Geometry: final body of the model. Coordinates: model frame, mm. Face numbers are marked on the shaded views. A direction names the side the tool comes from. Round coordinates to 2 decimals unless told otherwise and drop trailing zeros. Loops run counter-clockwise (first coordinate to the right, second up) from the corner with the lowest first, then second, coordinate; pieces in that order, holes last. Notation, with made-up numbers: M 57.25,53.25 L 111.25,53.25 A4 ccw 111.25,58.25 Z; hole C -12,14 d8. An arc over 180 degrees is marked long. Write each question's results on one line, items separated by ' | '.
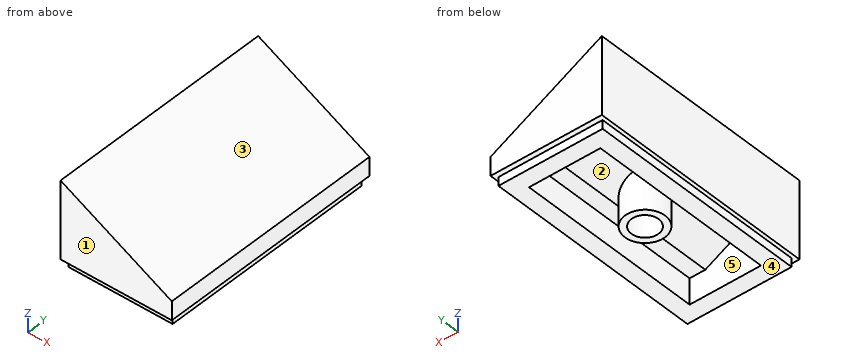
Solid Edge part; units mm, degrees
sketch "Sketch1" plane through (0, 0, 0) normal (0, 0, 1) x (1, 0, 0)
  line L0 (3.9, 7.9) -> (-3.9, 7.9)
  line L1 (-3.9, 7.9) -> (-3.9, -7.9)
  line L2 (-3.9, -7.9) -> (3.9, -7.9)
  line L3 (3.9, -7.9) -> (3.9, 7.9)
extrude "Protrusion1" add sketch "Sketch1" along normal blind 6
sketch "Sketch2" plane through (0, -7.9, 3) normal (0, -1, 0) x (1, 0, 0)
  line L0 (3.9, -3) -> (3.9, -1.1)
  line L1 (3.9, -1.1) -> (-3.9, 3)
  line L2 (-3.9, 3) -> (-3.9, 3.5621)
  line L3 (-3.9, 3.5621) -> (6.8698, 3.4105)
  line L4 (6.8698, 3.4105) -> (3.9, -3)
extrude "ExtrudedCutout_1" cut sketch "Sketch2" against normal blind 28.4067
sketch "Sketch3" plane through (0, 0, 0) normal (0, 0, -1) x (1, 0, 0)
  line L0 (3.65, 7.65) -> (-3.65, 7.65)
  line L1 (-3.65, 7.65) -> (-3.65, -7.65)
  line L2 (-3.65, -7.65) -> (3.65, -7.65)
  line L3 (3.65, -7.65) -> (3.65, 7.65)
  line L4 (-4.59, -8.7889) -> (5.3032, -8.7889)
  line L5 (5.3032, -8.7889) -> (5.3032, 8.7889)
  line L6 (5.3032, 8.7889) -> (-4.59, 8.7889)
  line L7 (-4.59, 8.7889) -> (-4.59, -8.7889)
extrude "ExtrudedCutout_2" cut sketch "Sketch3" against normal blind 0.6
sketch "Sketch4" plane through (0, 0, 0) normal (0, 0, -1) x (1, 0, 0)
  line L0 (-2.5, -6.5) -> (2.5, -6.5)
  line L1 (2.5, -6.5) -> (2.5, 6.5)
  line L2 (2.5, 6.5) -> (-2.5, 6.5)
  line L3 (-2.5, 6.5) -> (-2.5, -6.5)
extrude "ExtrudedCutout_3" cut sketch "Sketch4" against normal blind 1.8
sketch "Sketch5" plane through (0, 6.5, 0.9) normal (0, -1, 0) x (1, 0, 0)
  line L0 (-2.5, 0.9) -> (-2.5, 2.95)
  line L1 (1.4, 0.9) -> (-2.5, 2.95)
  line L2 (-2.5, 0.9) -> (1.4, 0.9)
extrude "Cutout1" cut sketch "Sketch5" along normal up to vertex (13 mm away)
sketch "Sketch6" plane through (0, 0, 0) normal (0, 0, -1) x (1, 0, 0)
  circle A0 centre (0, 0) radius 1.4
  circle A1 centre (0, 0) radius 0.95
extrude "ExtrudedProtrusion_2" add sketch "Sketch6" against normal blind 6.3788
sketch "Sketch7" plane through (0, -7.9, 3.3) normal (0, -1, 0) x (1, 0, 0)
  line L0 (-3.9, 2.7) -> (3.9, -1.4)
  line L1 (3.9, -1.4) -> (3.4688, 3.9064)
  line L2 (3.4688, 3.9064) -> (-3.9, 2.7)
extrude "ExtrudedCutout_5" cut sketch "Sketch7" against normal blind 34.0923
sketch "Sketch8" plane through (0, -7.9, 3.3) normal (0, -1, 0) x (0, 0, 1)
  line L0 (-2.7, -3.9) -> (-2.7, 3.9)
  line L1 (-2.7, 3.9) -> (2.7, 3.9)
  line L2 (2.7, 3.9) -> (-1.4, -3.9)
  line L3 (-1.4, -3.9) -> (-2.7, -3.9)
extrude "ExtrudedProtrusion_3" add sketch "Sketch8" along normal blind 0.1
sketch "Sketch9" plane through (0, 7.9, 3.3) normal (0, 1, 0) x (0, 0, -1)
  line L0 (-2.7, 3.9) -> (2.7, 3.9)
  line L1 (2.7, 3.9) -> (2.7, -3.9)
  line L2 (2.7, -3.9) -> (1.4, -3.9)
  line L3 (1.4, -3.9) -> (-2.7, 3.9)
extrude "ExtrudedProtrusion_4" add sketch "Sketch9" along normal blind 0.1
1. Section A-A (y = -5.75). Output: boundary loops of the cut face in (x, z), then the cut area to 3 significant figures.
Answer key:
outline: M -3.9,0.6 L -3.65,0.6 L -3.65,0 L -2.5,0 L -2.5,3.85 L 1.4,1.8 L 2.5,1.8 L 2.5,0 L 3.65,0 L 3.65,0.6 L 3.9,0.6 L 3.9,1.9 L -3.9,6 Z | area: 17.5 mm²
2. Section D-D (x = -0.5). Output: boundary loops of the cut face in (y, z).
Answer key:
outline: M -8,0.6 L -7.65,0.6 L -7.65,0 L -6.5,0 L -6.5,2.8 L -1.31,2.8 L -1.31,0 L -0.81,0 L -0.81,2.8 L 0.81,2.8 L 0.81,0 L 1.31,0 L 1.31,2.8 L 6.5,2.8 L 6.5,0 L 7.65,0 L 7.65,0.6 L 8,0.6 L 8,4.21 L -8,4.21 Z
3. Access query for the marked faces 4 and 5. Directions: +Z, -Z, +X, -X, +Y, -Y. A direction counts if a zero-diameter tool reaches every point of the face in a straight line with its end or side. Return the directions, or none.
Answer key:
face 4: -Z, +X, -X, +Y, -Y | face 5: -Z
4. Ray query, probe 1 along X at (y, z) = (0, 1.65); probe 2 along Y at (x, z) = (0, 1.5); probe 3 along Y at (x, z) = (-1.5, 1.4). Return the intervals inside material, ascending.
Answer key:
probe 1: x = -3.9 to -2.5, -1.4 to -0.95, 0.95 to 1.4, 2.5 to 3.9 | probe 2: y = -8 to -6.5, -1.4 to -0.95, 0.95 to 1.4, 6.5 to 8 | probe 3: y = -8 to -6.5, 6.5 to 8
5. Section C-C (z = 4.1). Output: boundary loops of the cut face in (x, y).
Answer key:
outline: M -3.9,-8 L -0.29,-8 L -0.29,8 L -3.9,8 Z
6. Section B-B (x = 0.75). Output: boundary loops of the cut face in (y, z).
Answer key:
outline: M -8,0.6 L -7.65,0.6 L -7.65,0 L -6.5,0 L -6.5,2.14 L -1.18,2.14 L -1.18,0 L -0.58,0 L -0.58,2.14 L 0.58,2.14 L 0.58,0 L 1.18,0 L 1.18,2.14 L 6.5,2.14 L 6.5,0 L 7.65,0 L 7.65,0.6 L 8,0.6 L 8,3.56 L -8,3.56 Z
7. Draft query along Y for the marked faces 1, 2 and 3. Return one class per face: pulls with the +Y half, pulls with the -Y half, needs draft (parallel to the pull), parting line crosses it, or undercut.
Answer key:
face 1: pulls with the -Y half | face 2: undercut | face 3: needs draft
8. Pin query (flat end, axial travel): P1, Ø0.5, axis at x = -1, z = 0.5, coming from the +Y side; P2, Ø1, axis at x = 1.5, y = -2.5, coming from the -Z side; P3, Ø1.5, axis at y = 2.5, z = 4.5, coming from the +X side; P4, Ø4, axis at x = 2.5, y = -5, coming from the +Z side. Return the tip coordinate at first contact, or that it passes through.
Answer key:
P1: stops at y = 8 | P2: stops at z = 1.8 | P3: stops at x = 0.38 | P4: stops at z = 3.69
